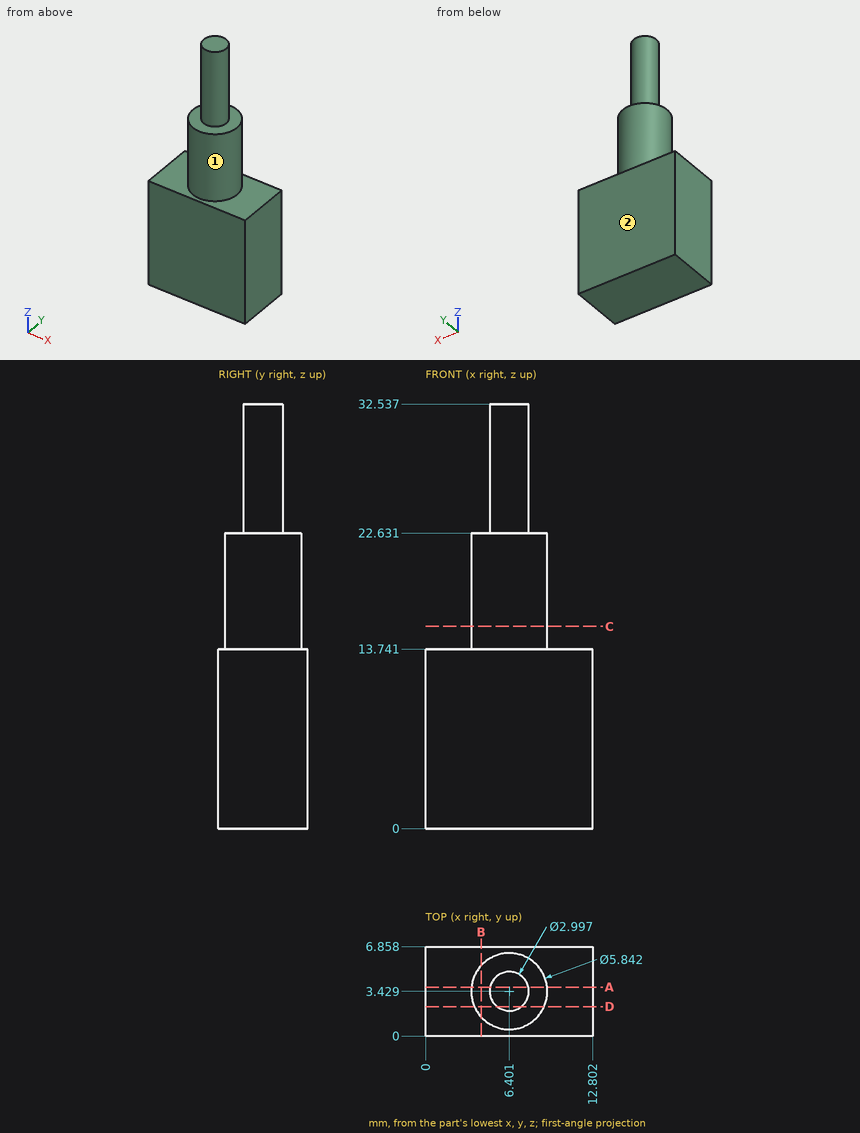
Geometry check sheet. Reference: drawing and pictorial views, mm from the part's lowest x, y, z. A direction names the side the tool comes from. Give positions to 0.01 mm unless a question says otherwise; leave off trailing zeros. Write each loop counter-clockwise with the first axis right and the second up, starting at its lowest first coordinate (ties: lowest second). Pieces come first, ordered by that corner, then holes. Notation, with made-up numbers: (39.25, 23.5) - (79.25, 23.5) arc R22 ccw to (79.25, 48.5) - close; hole circle Ø6 at (81, 60). An arc over 180 degrees is marked (long way). Put each result on its own line as item: value.
Q1. Section check D-D on y = 2.25. Record the cut outline in (x, z) (1 decimal).
Result:
outline: (0, 0) - (12.8, 0) - (12.8, 13.7) - (9.1, 13.7) - (9.1, 22.6) - (7.3, 22.6) - (7.3, 32.5) - (5.5, 32.5) - (5.5, 22.6) - (3.7, 22.6) - (3.7, 13.7) - (0, 13.7) - close
Q2. Depth check by flat-ended pin: P1, Ø1, axis at x = 5.5, z = 20.5, coming from the +Y side. Enter the tip coordinate at first touch or a pass-through.
Result:
P1: y = 6.32
Q3. Set-up check for the marked faces 1 and 2: record each of +Z, -Z, +X, -X, +Y, -Y from which the full face is reachable in a straight line by a thin tool's end or side.
Result:
face 1: +Z
face 2: +Z, -Z, +X, -X, +Y
Q4. Scan lines: probe 1 along Z at (x, y) = (1.25, 1.5); probe 2 along Z at (x, y) = (5.5, 5.75); probe 3 along X at (y, z) = (2.25, 17). Record each from-to range of solid material in increasing order. Write a range as from..to.
Result:
probe 1: 0..13.74
probe 2: 0..22.63
probe 3: 3.73..9.07
Q5. Section check B-B on x = 4.25. Record the cut outline in (y, z) (1 decimal).
Result:
outline: (0, 0) - (6.9, 0) - (6.9, 13.7) - (5.4, 13.7) - (5.4, 22.6) - (1.5, 22.6) - (1.5, 13.7) - (0, 13.7) - close
Q6. Section check A-A on y = 3.75. Record the cut outline in (x, z) (1 decimal).
Result:
outline: (0, 0) - (12.8, 0) - (12.8, 13.7) - (9.3, 13.7) - (9.3, 22.6) - (7.9, 22.6) - (7.9, 32.5) - (4.9, 32.5) - (4.9, 22.6) - (3.5, 22.6) - (3.5, 13.7) - (0, 13.7) - close
Q7. Section check C-C on z = 15.5. Record the cut outline in (x, y), and give its area (3 significant figures).
Result:
outline: circle Ø5.84 at (6.4, 3.43)
area: 26.8 mm2
